Verification items for the finished model (mm, model axes). A direction names the side the tool comes from. Coordinates: 2 decimals unless noted, no trailing zeros. Order: outer loops, then holes, each group sorted by start corner. A loop starts at its lowest first (then second) coordinate and runs counter-clockwise, first axis right, second up. Notation, with made-up numbers: (16, 88) - (28, 88) arc R18 cw to (28, 104) - close; hole circle Ø5 at (56.5, 7.25). An arc over 180 degrees is marked (long way). Answer as CSV lines item,"result". Start each with the question number.
1. Section check C-C (y = 29). Record the cut outline in (x, z), and give its area (3 significant figures).
2. Go/stop test with flat-tipped pins: pin 1 (5.5 mm diameter, centred on x = -64.5, y = 12, fed in from -Z); pin 2 (6.5 mm diameter, centred on x = 64, y = -26.61, fed in from +Z); pin 3 (7 mm diameter, centred on x = 16, y = -8.61, fed in from +Z). Record where each tip stops, or that it passes through.
3. Section check A-A (x = -16). Record the cut outline in (y, z), and give its area (3 significant figures).
4. Section check D-D (x = -64). Count the separate pieces of the cut face and the enclosed holes in it, and give its area (3 significant figures).
5. Set-up check for faces 3 (the cylindrical face through (-66.747, -26.487, 4.732)), 4 (the flat face through (23, 7, 7)), 5 (the flat face through (67, 12, 2.4)): record each of +Z, -Z, +X, -X, +Y, -Y from which the full face is reachable in a straight line by a thin tool's end or side.
6. Material ranges on L1, parallel to X at y = 1, z = 9.25; L2, parallel to Y at x = 36, z = 6; L3, parallel to X at y = -43.5, z = 2.5, recorded low to high. Write a range as [from, to].
7. Mould release check, pull along X, two halves, no side actions. Record for faces 1 (the flat face through (-28, 7, 10)), 2 (the cylindrical face through (61.97, 41.25, 4.73)): pulls with the +X half, pulls with the -X half, needs draft (parallel to the pull), parting line crosses it, or undercut.
8. Section check B-B (y = -46). Record the cut outline in (x, z), and give its area (3 significant figures).
from build123d import *

# Parameters (mm, degrees)
ESQUISSE1_W                                        = 148
ESQUISSE1_H                                        = 120
ESQUISSE1_R                                        = 2.5
ESQUISSE1_R_2                                      = 2
EXTRUSION1_DEPTH                                   = 4
ESQUISSE4_W                                        = 54
ESQUISSE4_H                                        = 80
BOSS_EXTRU_1_DEPTH                                 = 3
ESQUISSE6_W                                        = 148
ESQUISSE6_H                                        = 120
BOSS_EXTRU_2_DEPTH                                 = 3
CHAMBRAGE_POUR_VIS_T_TE_HEXAGONALE_M41_D           = 4.5
CHAMBRAGE_POUR_VIS_T_TE_HEXAGONALE_M41_CBORE_D     = 10
CHAMBRAGE_POUR_VIS_T_TE_HEXAGONALE_M41_CBORE_DEPTH = 4.4
CHAMBRAGE_POUR_VIS_T_TE_HEXAGONALE_M51_D           = 5.5
CHAMBRAGE_POUR_VIS_T_TE_HEXAGONALE_M51_CBORE_D     = 11
CHAMBRAGE_POUR_VIS_T_TE_HEXAGONALE_M51_CBORE_DEPTH = 5.4
ESQUISSE11_W                                       = 4
ESQUISSE11_H                                       = 80
BOSS_EXTRU_3_DEPTH                                 = 3
ESQUISSE3_R                                        = 4
ENL_V_MAT_EXTRU_2_DEPTH                            = 8


with BuildPart() as part:
    # Esquisse1 → Extrusion1 (new body)
    with BuildSketch(Plane.XY):
        with Locations((0, 6.392373056)):
            Rectangle(ESQUISSE1_W, ESQUISSE1_H)
        with Locations((-64, -0.607626944)):
            Circle(ESQUISSE1_R, mode=Mode.SUBTRACT)
        with Locations((-36, -0.607626944)):
            Circle(ESQUISSE1_R, mode=Mode.SUBTRACT)
        with Locations((-64, -26.607626944)):
            Circle(ESQUISSE1_R, mode=Mode.SUBTRACT)
        with Locations((-36, -26.607626944)):
            Circle(ESQUISSE1_R, mode=Mode.SUBTRACT)
        with Locations((36, -0.607626944)):
            Circle(ESQUISSE1_R, mode=Mode.SUBTRACT)
        with Locations((64, -0.607626944)):
            Circle(ESQUISSE1_R, mode=Mode.SUBTRACT)
        with Locations((36, -26.607626944)):
            Circle(ESQUISSE1_R, mode=Mode.SUBTRACT)
        with Locations((64, -26.607626944)):
            Circle(ESQUISSE1_R, mode=Mode.SUBTRACT)
        with Locations((64, 39.392373056)):
            Circle(ESQUISSE1_R, mode=Mode.SUBTRACT)
        with Locations((36, 39.392373056)):
            Circle(ESQUISSE1_R, mode=Mode.SUBTRACT)
        with Locations((16, 21.392373056)):
            Circle(ESQUISSE1_R_2, mode=Mode.SUBTRACT)
        with Locations((16, -8.607626944)):
            Circle(ESQUISSE1_R_2, mode=Mode.SUBTRACT)
        with Locations((-16, 21.392373056)):
            Circle(ESQUISSE1_R_2, mode=Mode.SUBTRACT)
        with Locations((-16, -8.607626944)):
            Circle(ESQUISSE1_R_2, mode=Mode.SUBTRACT)
        with Locations((64, 13.392373056)):
            Circle(ESQUISSE1_R, mode=Mode.SUBTRACT)
        with Locations((36, 13.392373056)):
            Circle(ESQUISSE1_R, mode=Mode.SUBTRACT)
        with Locations((-36, 39.392373056)):
            Circle(ESQUISSE1_R, mode=Mode.SUBTRACT)
        with Locations((-64, 39.392373056)):
            Circle(ESQUISSE1_R, mode=Mode.SUBTRACT)
        with Locations((-36, 13.392373056)):
            Circle(ESQUISSE1_R, mode=Mode.SUBTRACT)
        with Locations((-64, 13.392373056)):
            Circle(ESQUISSE1_R, mode=Mode.SUBTRACT)
    extrude(amount=EXTRUSION1_DEPTH)

    # Esquisse4 → Boss.-Extru.1 (add)
    with BuildSketch(Plane.XY.offset(4)):
        with Locations((-47, 6.392373056)):
            Rectangle(ESQUISSE4_W, ESQUISSE4_H)
        with Locations((47, 6.392373056)):
            Rectangle(ESQUISSE4_W, ESQUISSE4_H)
    extrude(amount=BOSS_EXTRU_1_DEPTH)

    # Esquisse6 → Boss.-Extru.2 (add)
    with BuildSketch(Plane(origin=(0, 0, 0), x_dir=(-1, 0, 0), z_dir=(0, 0, -1))):
        with Locations((0, 6.392373056)):
            Rectangle(ESQUISSE6_W, ESQUISSE6_H)
    extrude(amount=BOSS_EXTRU_2_DEPTH)

    # Chambrage pour vis à tête hexagonale M41 (through all)
    with Locations(Plane(origin=(0, 0, -3), x_dir=(-1, 0, 0), z_dir=(0, 0, -1))):
        with Locations((-16, 21.392373056), (16, 21.392373056), (16, -8.607626944), (-16, -8.607626944)):
            CounterBoreHole(CHAMBRAGE_POUR_VIS_T_TE_HEXAGONALE_M41_D / 2, CHAMBRAGE_POUR_VIS_T_TE_HEXAGONALE_M41_CBORE_D / 2, CHAMBRAGE_POUR_VIS_T_TE_HEXAGONALE_M41_CBORE_DEPTH)

    # Chambrage pour vis à tête hexagonale M51 (through all)
    with Locations(Plane(origin=(0, 0, -3), x_dir=(-1, 0, 0), z_dir=(0, 0, -1))):
        with Locations((-64, -0.607626944), (-36, -0.607626944), (-36, -26.607626944), (-64, -26.607626944), (36, -0.607626944), (64, -0.607626944), (64, -26.607626944), (36, -26.607626944), (64, 39.392373056), (64, 13.392373056), (36, 39.392373056), (36, 13.392373056), (-36, 39.392373056), (-64, 39.392373056), (-64, 13.392373056), (-36, 13.392373056)):
            CounterBoreHole(CHAMBRAGE_POUR_VIS_T_TE_HEXAGONALE_M51_D / 2, CHAMBRAGE_POUR_VIS_T_TE_HEXAGONALE_M51_CBORE_D / 2, CHAMBRAGE_POUR_VIS_T_TE_HEXAGONALE_M51_CBORE_DEPTH)

    # Esquisse11 → Boss.-Extru.3 (add)
    with BuildSketch(Plane.XY.offset(7)):
        with Locations((-28, 6.392373056)):
            Rectangle(ESQUISSE11_W, ESQUISSE11_H)
        with Locations((28, 6.392373056)):
            Rectangle(ESQUISSE11_W, ESQUISSE11_H)
        with Locations((-72, 6.392373056)):
            Rectangle(ESQUISSE11_W, ESQUISSE11_H)
        with Locations((72, 6.392373056)):
            Rectangle(ESQUISSE11_W, ESQUISSE11_H)
    extrude(amount=BOSS_EXTRU_3_DEPTH)

    # Esquisse3 → Enlèv. mat.-Extru.2 (cut, through all)
    with BuildSketch(Plane.XY.offset(4)):
        with Locations((-31, 56.392373056)):
            Circle(ESQUISSE3_R)
        with Locations((31, 56.392373056)):
            Circle(ESQUISSE3_R)
        with Locations((-31, -43.607626944)):
            Circle(ESQUISSE3_R)
        with Locations((31, -43.607626944)):
            Circle(ESQUISSE3_R)
    extrude(amount=-ENL_V_MAT_EXTRU_2_DEPTH, mode=Mode.SUBTRACT)


solid = part.part
Evaluation:
1,outline,"(-74, -3) - (74, -3) - (74, 10) - (70, 10) - (70, 7) - (30, 7) - (30, 10) - (26, 10) - (26, 7) - (20, 7) - (20, 4) - (-20, 4) - (-20, 7) - (-26, 7) - (-26, 10) - (-30, 10) - (-30, 7) - (-70, 7) - (-70, 10) - (-74, 10) - close"
1,area,"1,410 mm²"
2,pin 1,"stops at z = 2.4"
2,pin 2,"stops at z = 7"
2,pin 3,"stops at z = 4"
3,outline,"(-53.61, -3) - (-13.61, -3) - (-13.61, 1.4) - (-10.86, 1.4) - (-10.86, 4) - (-53.61, 4) - close; (-6.36, 1.4) - (-3.61, 1.4) - (-3.61, -3) - (16.39, -3) - (16.39, 1.4) - (19.14, 1.4) - (19.14, 4) - (-6.36, 4) - close; (23.64, 1.4) - (26.39, 1.4) - (26.39, -3) - (66.39, -3) - (66.39, 4) - (23.64, 4) - close"
3,area,"729 mm²"
4,separate pieces,"5"
4,enclosed holes,"0"
4,area,"741 mm²"
5,face 3,"+Z, -Z"
5,face 4,"+Z, +Y, -Y"
5,face 5,"-Z"
6,L1,"x = [-74, -70], [-30, -26], [26, 30], [70, 74]"
6,L2,"y = [-33.61, -29.36], [-23.86, -3.36], [2.14, 10.64], [16.14, 36.64], [42.14, 46.39]"
6,L3,"x = [-74, -35], [-27, 27], [35, 74]"
7,face 1,"needs draft"
7,face 2,"undercut"
8,outline,"(-74, -3) - (-34.21, -3) - (-34.21, 4) - (-74, 4) - close; (-27.79, -3) - (27.79, -3) - (27.79, 4) - (-27.79, 4) - close; (34.21, -3) - (74, -3) - (74, 4) - (34.21, 4) - close"
8,area,"946 mm²"
